from build123d import *

# Parameters (mm, degrees)
BOSS_EXTRUDE1_DEPTH = 1.5
SKETCH2_R           = 1.25
SKETCH2_W           = 2.5
SKETCH2_H           = 2.5
BOSS_EXTRUDE2_DEPTH = 6.5
CUT_EXTRUDE1_DEPTH  = 0.6


with BuildPart() as part:
    # Sketch1 → Boss-Extrude1 (new body)
    with BuildSketch(Plane(origin=(0, 0, 0), x_dir=(1, 0, 0), z_dir=(0, 1, 0))):
        Polygon((0, 0), (71, 14.38), (71, 110), (0, 110), align=None)
    extrude(amount=BOSS_EXTRUDE1_DEPTH)

    # Sketch2 → Boss-Extrude2 (add)
    with BuildSketch(Plane(origin=(0, 1.5, 0), x_dir=(1, 0, 0), z_dir=(0, 1, 0))):
        with Locations(Location((11.5, 4.879915247, 0), (0, 0, 270))):
            Circle(SKETCH2_R)
        with Locations(Location((59.5, 14.601605388, 0), (0, 0, 270))):
            Circle(SKETCH2_R)
        with Locations((11.25, 107.5)):
            Rectangle(SKETCH2_W, SKETCH2_H)
    extrude(amount=-BOSS_EXTRUDE2_DEPTH)

    # Sketch3 → Cut-Extrude1 (cut)
    with BuildSketch(Plane(origin=(0, 0, 0), x_dir=(-1, 0, 0), z_dir=(0, -1, 0))):
        Polygon((-66, 105), (-66, 18.468844579), (-5, 6.114196692), (-5, 105), align=None)
    extrude(amount=-CUT_EXTRUDE1_DEPTH, mode=Mode.SUBTRACT)


solid = part.part
Can you work these out from the model? Positions are in its coordinate system, mm. A direction names the side the tool comes from. Round coordinates to 2 decimals unless told otherwise and drop trailing zeros. Loops run counter-clockwise (first coordinate to the right, second up) from the corner with the lowest first, then second, coordinate; pieces in that order, holes last. Notation, with made-up numbers: (-32, 59) - (16, 59) arc R21 ccw to (16, 67) - close; hole circle Ø1 at (8.25, 25). An arc over 180 degrees is marked (long way). Write item = value, one per line. Start each with the question number.
(1) For P1, Ø1.2, axis at y = -2.5, z = -108, coming from the +X side; P2, Ø0.8, axis at x = 11, y = -3, coming from the +Z side; P3, Ø0.8, axis at x = 11, y = -3.5, coming from the -Z side, each with a flat end and sliding along its axis, tell me the tip position at first contact or that it passes through.
(2) If we mould it in two halves opening along Z, with no side actions, what happens to faces 1 (the face through (60, -5, -15)), 2 (the face through (35.93, 0.3, -12.38)), 3 (the face through (35, 0.74, -7.09))? For each: released by +Z, released by -Z, zero draft, split by the parting line, or undercut.
(3) If we section it at C-C (x = 48.5): Please give me the cut outline in (y, z).
(4) For faces 4 (the face through (36, 0.6, -56)), 5 (the face through (11, -2, -108.75)), 6 (the face through (10, -2, -107)), 7 (the face through (12.5, -2, -107)), which set-ups out of +Z, -Z, +X, -X, +Y, -Y let a thin tool reach every point of the face, with its end or its side?
(5) If we section it at D-D (x = 59.5): Please give me the cut outline in (y, z).
(6) If we section it at B-B (y = -3): Please give me the cut outline in (x, z).
(7) If I drill on probe 1 along X at (y, z) = (0.25, -54.5); probe 2 along Y at (x, z) = (15.5, -48); probe 3 along Z at (x, y) = (10.5, -4.5), over which ranges is the centre line in solid material (lowest first)? Write a range as [from, to].
(8) If we section it at A-A (z = -103): Please give me the cut outline in (x, y).
Ans:
q1.P1 = 12.5
q1.P2 = -3.63
q1.P3 = -108.75
q2.face_1 = zero draft
q2.face_2 = undercut
q2.face_3 = released by +Z
q3.outline = (0, -110) - (1.5, -110) - (1.5, -9.82) - (0, -9.82) - (0, -14.92) - (0.6, -14.92) - (0.6, -105) - (0, -105) - close
q4.face_4 = -Y
q4.face_5 = -Z, +X, -X, -Y
q4.face_6 = +Z, -Z, -X, -Y
q4.face_7 = -Z, +X, -Y
q5.outline = (-5, -15.85) - (0, -15.85) - (0, -17.15) - (0.6, -17.15) - (0.6, -105) - (0, -105) - (0, -110) - (1.5, -110) - (1.5, -12.05) - (0, -12.05) - (0, -13.35) - (-5, -13.35) - close
q6.outline = (10, -108.75) - (12.5, -108.75) - (12.5, -106.25) - (10, -106.25) - close; circle Ø2.5 at (11.5, -4.88); circle Ø2.5 at (59.5, -14.6)
q7.probe_1 = [0, 5], [66, 71]
q7.probe_2 = [0.6, 1.5]
q7.probe_3 = [-108.75, -106.25], [-5.63, -4.13]
q8.outline = (0, 0) - (5, 0) - (5, 0.6) - (66, 0.6) - (66, 0) - (71, 0) - (71, 1.5) - (0, 1.5) - close
